```python
from build123d import *

# Parameters (mm, degrees)
SKETCH_1_R          = 19
EXTRUDE_1_DEPTH     = 2
SKETCH_2_R          = 19
SKETCH_2_R_2        = 15.9
EXTRUDE_2_DEPTH     = 8
SKETCH_3_R          = 11.5
CUT_EXTRUDE_1_DEPTH = 6


with BuildPart() as part:
    # 草图1 → 凸台-拉伸1 (new body)
    with BuildSketch(Plane(origin=(0, 0, 0), x_dir=(1, 0, 0), z_dir=(0, 1, 0))):
        with Locations(Location((0, 0, 0), (0, 0, 270))):
            Circle(SKETCH_1_R)
    extrude(amount=EXTRUDE_1_DEPTH)

    # 草图2 → 凸台-拉伸2 (add)
    with BuildSketch(Plane(origin=(0, 2, 0), x_dir=(1, 0, 0), z_dir=(0, 1, 0))):
        with Locations(Location((0, 0, 0), (0, 0, 270))):
            Circle(SKETCH_2_R)
        with Locations(Location((0, 0, 0), (0, 0, 270))):
            Circle(SKETCH_2_R_2, mode=Mode.SUBTRACT)
    extrude(amount=EXTRUDE_2_DEPTH)

    # 草图3 → 切除-拉伸1 (cut)
    with BuildSketch(Plane.XZ):
        with Locations(Location((0, 0, 0), (0, 0, 270))):
            Circle(SKETCH_3_R)
    extrude(amount=-CUT_EXTRUDE_1_DEPTH, mode=Mode.SUBTRACT)

    # 草图10 → M3 螺纹孔1 (revolve, cut)
    with BuildSketch(Plane(origin=(-19, 6.5, 0), x_dir=(0, 0, 1), z_dir=(0, 1, 0))):
        Polygon((0, 0), (0, 44.651075774), (1.25, 43.9), (1.25, 0.275), (1.525, 0), align=None)
    revolve(axis=Axis((-25.35, 6.5, 0), (1, 0, 0)), mode=Mode.SUBTRACT)


solid = part.part
```
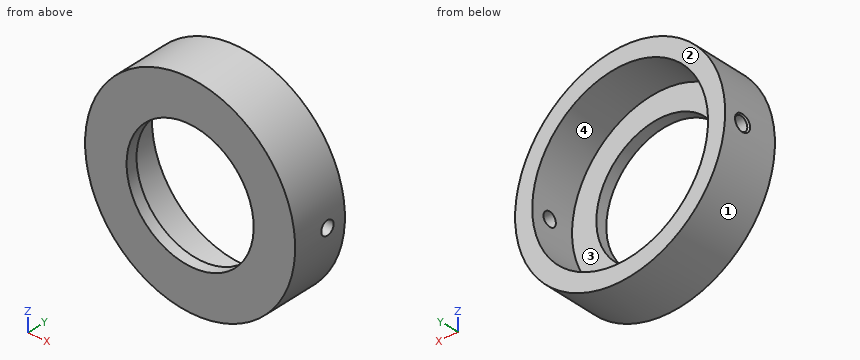
Design review of the part built by this model. Coordinates are the model's own, in mm. Face numbers are marked on the shaded views. Coordinates: 2 decimals unless noted, no trailing zeros. Order: outer loops, then holes, each group sorted by start corner. A loop starts at its lowest first (then second) coordinate and runs counter-clockwise, first axis right, second up.
1) Clearance check with flat-ended pins moving along their axes: pin 1 (5 mm diameter, centred on y = 5, z = -15, fed in from -X); pin 2 (5 mm diameter, centred on x = 5.5, y = 7, fed in from -Z); pin 3 (1.5 mm diameter, centred on y = 6, z = -4.5, fed in from +X). State where each tip first meets the part, or that it passes through.
2) Wall thickness on line 1 along X through (y, z) = (1.5, 0); line 2 along Y through (x, z) = (-16.75, 0); line 3 along X through (y, z) = (2.5, 13): over which ranges is each line inside the solid? List them lowest first.
3) Mouldability with a two-part tool opening along Z and no side actions: class the marked faces 1, 2, 3 and 4 as +Z half, -Z half, draft (parallel to the pull), parting line (faces both ways), or undercut.
4) Take a section at D-D, the plane y = 6.5. Give the boundary of the cut face in (x, z) (3 decimals).
5) Take a section at C-C, the plane z = -9.5. Give the boundary of the cut face in (x, y).
6) Take a section at B-B, the plane z = 0. Give the boundary of the cut face in (x, y) (3 decimals), and give its area (3 significant figures).
7) Take a section at A-A, the plane x = 0. Give the boundary of the cut face in (y, z), and give its area (3 significant figures).
Returned:
1. pin 1: stops at x = -14.31
1. pin 2: stops at z = -18.76
1. pin 3: stops at x = 18.63
2. line 1: x = -19 to -11.5, 11.5 to 19
2. line 2: y = 0 to 5.25, 7.75 to 10
2. line 3: x = -13.86 to -9.15, 9.15 to 13.86
3. face 1: parting line
3. face 2: draft
3. face 3: undercut
3. face 4: undercut
4. outline: (-18.943, -1.468) arc R19 ccw to (18.959, -1.25) - (15.851, -1.25) arc R15.9 cw to (-15.851, -1.25) - (-18.725, -1.25) - close; (-18.943, 1.468) - (-18.725, 1.25) - (-15.851, 1.25) arc R15.9 cw to (15.851, 1.25) - (18.959, 1.25) arc R19 ccw to start
5. outline: (-16.45, 0) - (-6.48, 0) - (-6.48, 2) - (-12.75, 2) - (-12.75, 10) - (-16.45, 10) - close; (6.48, 0) - (16.45, 0) - (16.45, 10) - (12.75, 10) - (12.75, 2) - (6.48, 2) - close
6. outline: (-19, 0) - (-11.5, 0) - (-11.5, 2) - (-15.9, 2) - (-15.9, 5.25) - (-18.725, 5.25) - (-19, 4.975) - close; (-19, 8.025) - (-18.725, 7.75) - (-15.9, 7.75) - (-15.9, 10) - (-19, 10) - close; (11.5, 0) - (19, 0) - (19, 5.25) - (15.9, 5.25) - (15.9, 2) - (11.5, 2) - close; (15.9, 7.75) - (19, 7.75) - (19, 10) - (15.9, 10) - close
6. area: 64.0 mm2
7. outline: (0, -19) - (10, -19) - (10, -15.9) - (2, -15.9) - (2, -11.5) - (0, -11.5) - close; (0, 11.5) - (2, 11.5) - (2, 15.9) - (10, 15.9) - (10, 19) - (0, 19) - close
7. area: 79.6 mm2
